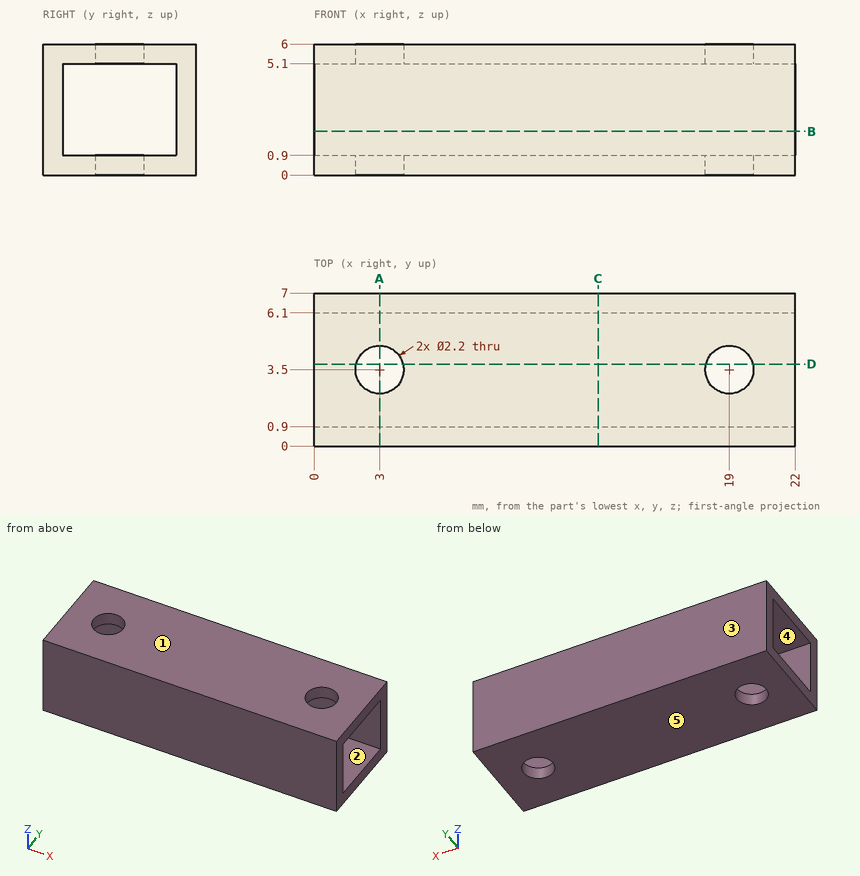
The drawing under review shows one solid part. Ordinate dimensions are in mm from its lowest x, y, z. A direction names the side the tool comes from. Round coordinates to 2 decimals unless told otherwise and drop trailing zeros. Loops run counter-clockwise (first coordinate to the right, second up) from the corner with the lowest first, then second, coordinate; pieces in that order, holes last. Notation, with made-up numbers: (35.25, 69.25) - (62.25, 69.25) arc R24 ccw to (62.25, 87.25) - close; hole circle Ø6 at (22, 46.25). An arc over 180 degrees is marked (long way). One line per question, with ' | ' between items.
1. Clearance check with a flat-ended pin moving along its axis: P1, Ø1.8, axis at x = 3, y = 3.5, coming from the -Z side. State where the tip first meets the part, or that it passes through.
Results are:
P1: passes through
2. Draft analysis for pull direction Z (two halves, no side actions). For the marked faces 1, 2 and 3, state which applies: released by +Z, released by -Z, zero draft, split by the parting line, or undercut.
Results are:
face 1: released by +Z | face 2: undercut | face 3: zero draft
3. We need section D-D, the plane y = 3.75. State the section outline as (x, z) points.
Results are:
outline: (0, 0) - (1.93, 0) - (1.93, 0.9) - (0, 0.9) - close; (0, 5.1) - (1.93, 5.1) - (1.93, 6) - (0, 6) - close; (4.07, 0) - (17.93, 0) - (17.93, 0.9) - (4.07, 0.9) - close; (4.07, 5.1) - (17.93, 5.1) - (17.93, 6) - (4.07, 6) - close; (20.07, 0) - (22, 0) - (22, 0.9) - (20.07, 0.9) - close; (20.07, 5.1) - (22, 5.1) - (22, 6) - (20.07, 6) - close
4. We need section B-B, the plane z = 2. State the section outline as (x, y) points, and give its area (3 significant figures).
Results are:
outline: (0, 0) - (22, 0) - (22, 0.9) - (0, 0.9) - close; (0, 6.1) - (22, 6.1) - (22, 7) - (0, 7) - close | area: 39.6 mm²
5. For L1, parallel to Z at x = 1.5, y = 1; L2, parallel to Y at x = 19, z = 5.3; L3, parallel to Y at x = 18, z = 4.55, list the stretches that pass through material, from the lowest coordinate up. Write a range as [from, to].
Results are:
L1: z = [0, 0.9], [5.1, 6] | L2: y = [0, 2.4], [4.6, 7] | L3: y = [0, 0.9], [6.1, 7]
6. We need section A-A, the plane x = 3. State the section outline as (y, z) points, and give its area (3 significant figures).
Results are:
outline: (0, 0) - (2.4, 0) - (2.4, 0.9) - (0.9, 0.9) - (0.9, 5.1) - (2.4, 5.1) - (2.4, 6) - (0, 6) - close; (4.6, 0) - (7, 0) - (7, 6) - (4.6, 6) - (4.6, 5.1) - (6.1, 5.1) - (6.1, 0.9) - (4.6, 0.9) - close | area: 16.2 mm²
7. We need section C-C, the plane x = 13. State the section outline as (y, z) points, and give its area (3 significant figures).
Results are:
outline: (0, 0) - (7, 0) - (7, 6) - (0, 6) - close; hole (0.9, 0.9) - (6.1, 0.9) - (6.1, 5.1) - (0.9, 5.1) - close | area: 20.2 mm²
8. For the marked faces 4 and 5, list the 3-axis set-ups (+Z, -Z, +X, -X, +Y, -Y) from which the entire face can be reached by the end or side of a thin tool; tool diameter is ignored.
Results are:
face 4: +X, -X | face 5: -Z, +X, -X, +Y, -Y
